Autodesk Inventor part; units mm, degrees
ref_plane "YZ Plane" through (0, 0, 0) normal (1, 0, 0) x (0, 1, 0)
ref_plane "XZ Plane" through (0, 0, 0) normal (0, 1, 0) x (-1, 0, 0)
ref_plane "XY Plane" through (0, 0, 0) normal (0, 0, 1) x (1, 0, 0)
sketch "Sketch1" plane through (0, 0, 0) normal (0, 0, 1) x (1, 0, 0)
  circle A0 centre (0, 0) radius 3
  dimension "d0" = 6
extrude "Extrusion1" add sketch "Sketch1" along normal blind 12
sketch "Sketch2" plane through (0, 0, 0) normal (0, 0, -1) x (-1, 0, 0)
  circle A0 centre (0, 0) radius 3
  circle A1 centre (0, 0) radius 5
  dimension "d3" = 10
extrude "Extrusion2" add sketch "Sketch2" along normal blind 6 contours A0 | A1
sketch "Sketch3" plane through (0, 0, -6) normal (0, 0, -1) x (-1, 0, 0)
  circle A0 centre (0, 0) radius 5
  line L0 (-1.4434, 2.5) -> (1.4434, 2.5)
  line L1 (1.4434, 2.5) -> (2.8868, 0)
  line L2 (2.8868, 0) -> (1.4434, -2.5)
  line L3 (1.4434, -2.5) -> (-1.4434, -2.5)
  line L4 (-1.4434, -2.5) -> (-2.8868, 0)
  line L5 (-2.8868, 0) -> (-1.4434, 2.5)
  dimension "d6" = 5
extrude "Extrusion3" cut sketch "Sketch3" against normal blind 3 contours L0 L1 L2 L3 L4 L5
thread "Thread1"
chamfer "Chamfer1" distance 0.508 angle 45 3 edges at (5, 0, -6) (5, 0, 0) (-3, 0, 12)
properties part number "M6 x 12mm" material "Steel"
Input: part model. Units: mm. Frame: model coordinates. A direction names the side the tool comes from. Give positions to 0.01 mm unless a question says otherwise; leave off trailing zeros. Write each loop counter-clockwise with the first axis right and the second up, starting at its lowest first coordinate (ties: lowest second). Pieces come first, ordered by that corner, then holes.
Q1. Section A-A, the plane x = 0. Output: boundary loops of the cut face in (y, z).
Q2. Set-up query: faces 4 (the face through (-3, 0, 6)), 5 (the face through (0, 0, 12)), 6 (the face through (2.155, -1.267, -4.521)). Return all of +Z, -Z, +X, -X, +Y, -Y with unobstructed straight access to the full face (end or side cutting, diameter ignored); none if empty.
Q3. Material intervals for probe 1 along Z at (x, y) = (-0.5, 4); probe 2 along Y at (x, z) = (-1, -4.5); probe 3 along Z at (x, y) = (1.5, 0.75), sorted ascending.
Q4. Section B-B, the plane z = 3.75. Output: boundary loops of the cut face in (x, y).
Q5. First-contact query: P1, Ø2, axis at y = 1.5, z = 9.5, coming from the +X side; P2, Ø1.5, axis at x = -2, z = 0, coming from the -Y side. Flat tips, straight axial feed; report the tip coordinate or a pass-through.
Q6. Section C-C, the plane z = -1. Output: boundary loops of the cut face in (x, y).
Q7. Pull-direction query (X, two-part tool) for faces 1 (the face through (-2, -2, -6)), 2 (the face through (1.08, 4.88, -2.97)), 3 (the face through (0, 2.5, -5)); classes: pulls with the +X half, pulls with the -X half, needs draft (parallel to the pull), parting line crosses it, or undercut.
Filled in:
1. outline: (-5, -5.49) - (-4.49, -6) - (-2.5, -6) - (-2.5, -3) - (2.5, -3) - (2.5, -6) - (4.49, -6) - (5, -5.49) - (5, -0.51) - (4.49, 0) - (3, 0) - (3, 11.49) - (2.49, 12) - (-2.49, 12) - (-3, 11.49) - (-3, 0) - (-4.49, 0) - (-5, -0.51) - close
2. face 4: +Z
2. face 5: +Z, +X, -X, +Y, -Y
2. face 6: -Z
3. probe 1: z = -6 to 0
3. probe 2: y = -4.9 to -2.5, 2.5 to 4.9
3. probe 3: z = -3 to 12
4. outline: circle Ø6 at (0, 0)
5. P1: stops at x = 2.96
5. P2: stops at y = -4.79
6. outline: circle Ø10 at (0, 0)
7. face 1: needs draft
7. face 2: parting line crosses it
7. face 3: undercut
